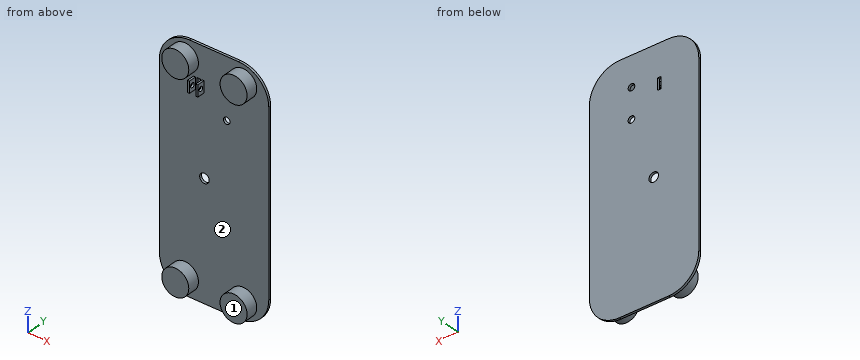
Autodesk Inventor part; units mm, degrees
ref_plane "YZ Plane" through (0, 0, 0) normal (1, 0, 0) x (0, 1, 0)
ref_plane "XZ Plane" through (0, 0, 0) normal (0, 1, 0) x (-1, 0, 0)
ref_plane "XY Plane" through (0, 0, 0) normal (0, 0, 1) x (1, 0, 0)
sketch "Sketch1" plane through (0, 0, 0) normal (0, 1, 0) x (-1, 0, 0)
  line L0 (-25.2222, 0) -> (-46.0502, 0)
  line L1 (-58.7502, -12.7) -> (-58.7502, -88.8746)
  line L2 (-46.0502, -101.5746) -> (-25.2222, -101.5746)
  line L3 (-12.5222, -88.8746) -> (-12.5222, -12.7)
  arc A0 (-12.5222, -12.7) -> (-25.2222, 0) centre (-25.2222, -12.7) ccw
  arc A1 (-46.0502, 0) -> (-58.7502, -12.7) centre (-46.0502, -12.7) ccw
  arc A2 (-58.7502, -88.8746) -> (-46.0502, -101.5746) centre (-46.0502, -88.8746) ccw
  arc A3 (-25.2222, -101.5746) -> (-12.5222, -88.8746) centre (-25.2222, -88.8746) ccw
  circle A4 centre (-31.5722, -52.0446) radius 2.0066
  line L4 (-28.3972, -13.5636) -> (-29.8704, -13.5636)
  line L5 (-28.3972, -13.5636) -> (-28.3972, -18.4404)
  line L6 (-28.3972, -18.4404) -> (-29.8704, -18.4404)
  line L7 (-29.8704, -18.4404) -> (-29.8704, -13.5636)
  circle A5 centre (-40.9702, -12.7) radius 1.4097
  circle A6 centre (-40.9702, -25.4) radius 1.4097
  point P0 (0, 0)
  dimension "d1" = 101.5746
  dimension "d2" = 12.7
  dimension "d3" = 12.7
  dimension "d4" = 12.7
  dimension "d5" = 12.7
  dimension "d6" = 12.7
  dimension "d7" = 12.7
  dimension "d8" = 12.7
  dimension "d9" = 12.7
  dimension "d10" = 46.228
  dimension "d11" = 19.05
  dimension "d12" = 49.53
  dimension "d13" = 4.0132
  dimension "d14" = 1.4732
  dimension "d15" = 13.5636
  dimension "d16" = 4.8768
  dimension "d17" = 15.875
  dimension "d18" = 12.7
  dimension "d19" = 17.78
  dimension "d20" = 12.7
  dimension "d21" = 2.8194
  dimension "d22" = 2.8194
extrude "Extrusion1" add sketch "Sketch1" along normal blind 0.9779
sketch "Sketch2" plane through (0, 0, 0) normal (0, -1, 0) x (1, 0, 0)
  line L0 (58.7502, -88.8746) -> (58.7502, -12.7)
  line L1 (46.0502, 0) -> (25.2222, 0)
  circle A0 centre (47.9552, -7.62) radius 5.715
  line L2 (12.5222, -12.7) -> (12.5222, -88.8746)
  circle A1 centre (23.3172, -7.62) radius 5.715
  line L3 (25.2222, -101.5746) -> (46.0502, -101.5746)
  circle A2 centre (47.9552, -93.9546) radius 5.715
  circle A3 centre (23.3172, -93.9546) radius 5.715
  line L4 (29.8704, -13.5636) -> (29.8704, -18.4404)
  line L5 (31.1404, -17.3228) -> (33.274, -17.3228)
  line L6 (33.274, -17.3228) -> (33.274, -22.1996)
  line L7 (33.274, -22.1996) -> (31.1404, -22.1996)
  line L8 (31.1404, -22.1996) -> (31.1404, -17.3228)
  line L9 (29.8704, -13.5636) -> (28.3972, -13.5636)
  line L10 (29.8704, -18.4404) -> (28.3972, -18.4404)
  line L11 (25.0952, -17.3228) -> (22.9616, -17.3228)
  line L12 (22.9616, -17.3228) -> (22.9616, -22.1996)
  line L13 (22.9616, -22.1996) -> (25.0952, -22.1996)
  line L14 (25.0952, -22.1996) -> (25.0952, -17.3228)
  point P0 (0, 0)
  dimension "d25" = 10.795
  dimension "d26" = 7.62
  dimension "d27" = 11.43
  dimension "d28" = 10.795
  dimension "d29" = 11.43
  dimension "d30" = 7.62
  dimension "d31" = 11.43
  dimension "d32" = 11.43
  dimension "d33" = 1.27
  dimension "d34" = 2.1336
extrude "Extrusion2" add sketch "Sketch2" along normal blind 5.08 contours A0 | A1 | A2 | A3
sketch "Sketch3" plane through (0, 0, 0) normal (0, -1, 0) x (1, 0, 0)
  line L0 (30.5054, -13.5636) -> (31.3218, -13.5636)
  line L1 (31.3218, -13.5636) -> (31.3218, -18.4404)
  line L2 (31.3218, -18.4404) -> (30.5054, -18.4404)
  line L3 (30.5054, -18.4404) -> (30.5054, -13.5636)
  line L4 (29.8704, -13.5636) -> (29.8704, -18.4404)
  line L5 (28.3972, -18.4404) -> (28.3972, -13.5636)
  line L6 (29.1338, -12.4667) -> (29.1338, -19.0142)
  line L7 (27.7622, -13.5636) -> (26.9458, -13.5636)
  line L8 (26.9458, -13.5636) -> (26.9458, -18.4404)
  line L9 (26.9458, -18.4404) -> (27.7622, -18.4404)
  line L10 (27.7622, -18.4404) -> (27.7622, -13.5636)
  point P0 (0, 0)
  dimension "d37" = 0.635
  dimension "d38" = 1.4732
  dimension "d39" = 0.7366
extrude "Extrusion3" add sketch "Sketch3" along normal blind 3.175
sketch "Sketch4" plane through (26.9458, 0, -18.4404) normal (-1, 0, 0) x (0, 0, 1)
  line L0 (0, 0) -> (0, -3.175)
  line L1 (4.8768, 0) -> (4.8768, -3.175)
  line L2 (4.8768, -3.175) -> (0, -3.175)
  line L3 (5.7404, 0) -> (-70.4342, 0)
  circle A0 centre (2.4384, -1.5875) radius 0.9525
  point P0 (18.4404, 0)
  dimension "d42" = 2.4384
  dimension "d43" = 4.8768
  dimension "d44" = 1.5875
  dimension "d45" = 3.175
  dimension "d46" = 1.905
extrude "Extrusion4" cut sketch "Sketch4" against normal through all contours A0
properties part number "base" material "Aluminum 6061"
Verification items for the finished model (mm, model axes). Face numbers are marked on the shaded views. Give positions to 0.01 mm unless a question says otherwise; leave off trailing zeros. Order: outer loops, then holes, each group sorted by start corner. A loop starts at its lowest first (then second) coordinate and runs counter-clockwise, first axis right, second up. Notation, with made-up numbers: M 58,43.25 L 69,43.25 A16 cw 69,66.25 Z; hole C 46.5,-29 d7. An arc over 180 degrees is marked long. Return JSON: item names as keys, results as strings. Group by question number.
1) Go/stop test with flat-tipped pins: pin 1 Ø3 at (x, y) = (32, -4) entering from -Z; pin 2 Ø2.5 at (x, z) = (40.97, -25.4) entering from +Y; pin 3 Ø1 at (x, y) = (28, -3.5) entering from +Z; pin 4 Ø2.5 at (y, z) = (-1.5, -15.5) entering from -X. Record where each tip stops, or that it passes through.
2) Section check B-B on z = -9. Record the cut outline in (x, y), and give its area (3 significant figures).
3) Mould release check, pull along Z, two halves, no side actions. Record for the marked faces 1 and 2: pulls with the +Z half, pulls with the -Z half, needs draft (parallel to the pull), parting line crosses it, or undercut.
4) Section check A-A on z = -25.4. Record the cut outline in (x, y), and give its area (3 significant figures).
5) Scan lines: line 1 (Y direction, x = 37, z = -64.5); line 2 (Z direction, x = 21, y = -4.25); line 3 (Z direction, x = 43, y = -1.5). Record each from-to range of solid material in increasing order.
6) Section check C-C on z = -69. Record the cut outline in (x, y), and give its area (3 significant figures).
Answer block:
{
 "1": {"pin 1": "stops at z = -18.44", "pin 2": "passes through", "pin 3": "stops at z = -3.73", "pin 4": "stops at x = 26.95"},
 "2": {"outline": "M 13.07,0 L 17.77,0 L 17.77,-5.08 L 28.86,-5.08 L 28.86,0 L 42.41,0 L 42.41,-5.08 L 53.5,-5.08 L 53.5,0 L 58.2,0 L 58.2,0.98 L 13.07,0.98 Z", "area": "157 mm^2"},
 "3": {"face 1": "needs draft", "face 2": "undercut"},
 "4": {"outline": "M 12.52,0 L 39.56,0 L 39.56,0.98 L 12.52,0.98 Z; M 42.38,0 L 58.75,0 L 58.75,0.98 L 42.38,0.98 Z", "area": "42.4 mm^2"},
 "5": {"line 1": "y = 0 to 0.98", "line 2": "z = -99.18 to -88.73, -12.84 to -2.4", "line 3": "z = -96.8 to -91.11, -10.47 to -4.77"},
 "6": {"outline": "M 12.52,0 L 58.75,0 L 58.75,0.98 L 12.52,0.98 Z", "area": "45.2 mm^2"}
}
